Can you work these out from the drawing? Everything is in mm from the part's minimum corner. A direction names the side the tool comes from. Give positions to 0.01 mm unless a question says otherwise; leave off trailing zeros. Order: outer loops, then holes, each group sorted by start corner. A loop starts at its lowest first (then second) coordinate and runs counter-clockwise, first axis right, second up. Notation, with made-up numbers: (-28, 26.25) - (17, 26.25) arc R25 cw to (17, 47.25) - close; hole circle Ø6 at (44.25, -25). An arc over 180 degrees is marked (long way). Write each question's results on one line, items separated by ' | '. Start each with the question number.
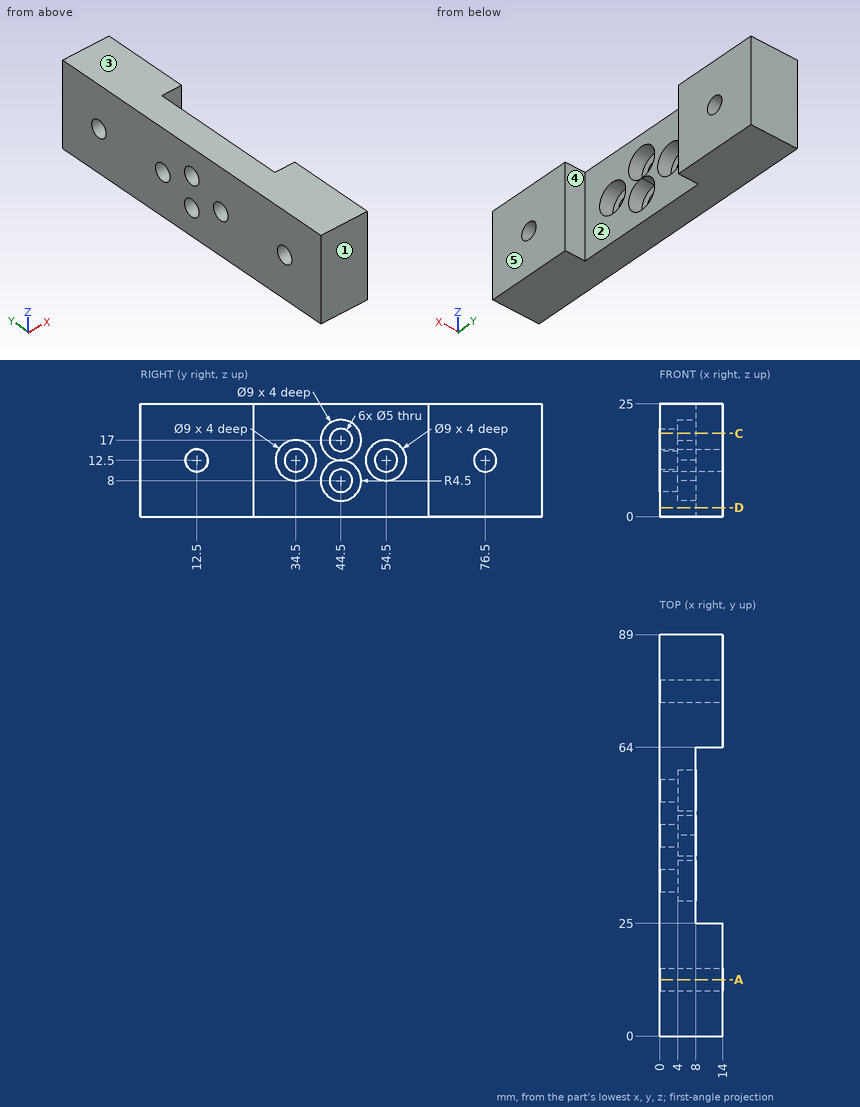
Q1. Thinking about a two-plate mould opening in Y: for the marked faces 1, 2 and 3, which applies, released by +Y, released by -Y, zero draft, split by the parting line, or undercut?
Q2. If we section it at C-C (z = 18.5): Please give me the cut outline in (x, y).
Q3. If we section it at A-A (y = 12.5): Please give me the cut outline in (x, z).
Q4. If I drill on probe 1 along Y at (x, z) = (2.25, 12.25); probe 2 along Y at (x, z) = (9.5, 12.5); probe 3 along Y at (x, z) = (2.25, 8), over which ranges is the centre line in solid material (lowest first)? Write a range as from..to.
Q5. Will these pins go through, and if not, where does the flat tip stop? P1, Ø10, axis at y = 32.5, z = 14, coming from the +X side; P2, Ø8, axis at y = 44.5, z = 8, coming from the +X side.
Q6. Which directions (+Z, -Z, +X, -X, +Y, -Y) give clear straight access to the entire face, cutting with the end or side of a thin tool? Please do the marked faces 4 and 5.
Q7. If we section it at D-D (z = 2): Please give me the cut outline in (x, y), plus the area to 3 significant figures.
Findings below:
1) face 1: released by -Y | face 2: undercut | face 3: zero draft
2) outline: (0, 0) - (14, 0) - (14, 25) - (8, 25) - (8, 40.26) - (4, 40.26) - (4, 42.5) - (0, 42.5) - close; (0, 46.5) - (4, 46.5) - (4, 48.74) - (8, 48.74) - (8, 64) - (14, 64) - (14, 89) - (0, 89) - close
3) outline: (0, 0) - (14, 0) - (14, 10) - (0, 10) - close; (0, 15) - (14, 15) - (14, 25) - (0, 25) - close
4) probe 1: y = 0..10.01, 14.99..32.01, 36.99..52.01, 56.99..74.01, 78.99..89 | probe 2: y = 0..10, 15..25, 64..74, 79..89 | probe 3: y = 0..42, 47..89
5) P1: stops at x = 8 | P2: stops at x = 4
6) face 4: +Z, -Z, +X | face 5: +Z, -Z, +X, +Y, -Y
7) outline: (0, 0) - (14, 0) - (14, 25) - (8, 25) - (8, 64) - (14, 64) - (14, 89) - (0, 89) - close | area: 1,010 mm2
